Study the drawing (mm; zero at the part's minimum x, y, z) and answer. Coordinates: 2 decimals unless noted, no trailing zeros. Write each question's results on one line, items separated by ' | '. Start each with the question number.
(1) Given pin 1 (6 mm diameter, centred on x = 60.32, y = 17.46, fed in from -Z), flat-ended and moving along its own axis, determine where the tip first touches the part or whether it passes through.
(2) The part is cut by section A-A, the plane z = 3.5. Count the separate pieces of the cut face and the enclosed holes in it, then the cut area to 3 significant figures.
(3) Determine the mould class of the marked faces 1, 2, 3 and 4 for opening direction Y: +Y half, -Y half, draft (parallel to the pull), parting line (faces both ways), or undercut.
(4) Straight lines are drawn through the part: L1, parallel to X at y = 18, z = 1.75; L2, parallel to Y at x = 65, z = 1.75 (1 decimal). For each, find the intervals that lie inside material, in ascending order.
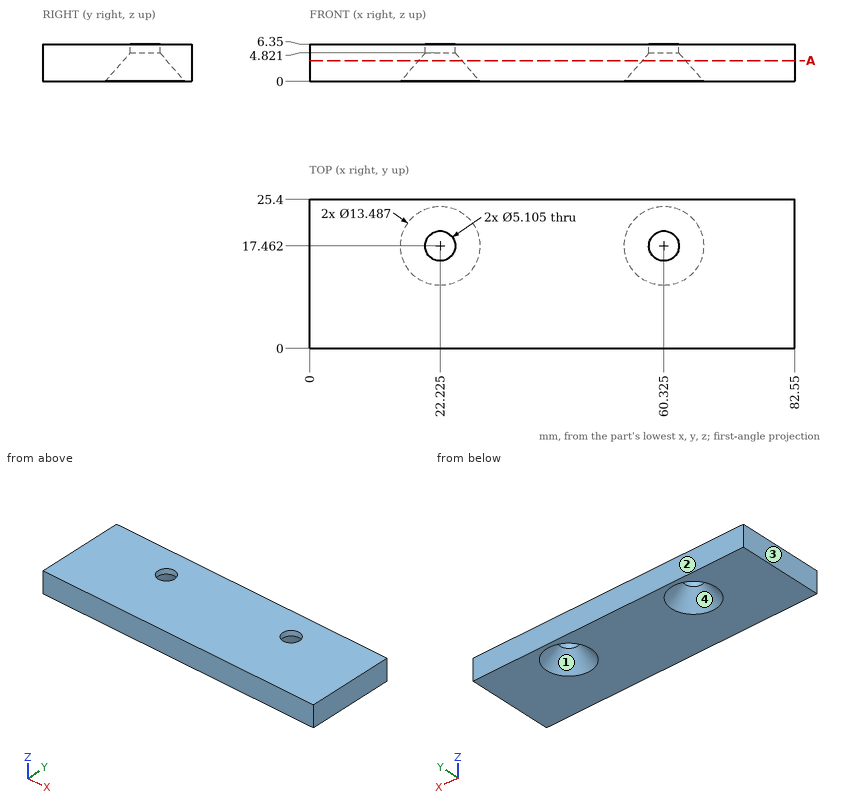
Established:
1) pin 1: stops at z = 4.3
2) separate pieces: 1 | enclosed holes: 2 | area: 2,010 mm^2
3) face 1: undercut | face 2: +Y half | face 3: draft | face 4: undercut
4) L1: x = 0 to 17.03, 27.42 to 55.13, 65.52 to 82.55 | L2: y = 0 to 15.1, 19.8 to 25.4
